The drawing under review shows one solid part. Ordinate dimensions are in mm from its lowest x, y, z. A direction names the side the tool comes from. Give positions to 0.01 mm unless a question says otherwise; leave off trailing zeros. Order: outer loops, then holes, each group sorted by start corner. A loop starts at its lowest first (then second) coordinate and runs counter-clockwise, first axis right, second up. Notation, with made-up numbers: (65, -16) - (95, -16) arc R20 ccw to (95, 5) - close; hole circle Ø6 at (53.25, -27.5). An arc over 180 degrees is marked (long way). Answer as a JSON object with one key per item and string values. Group by question number.
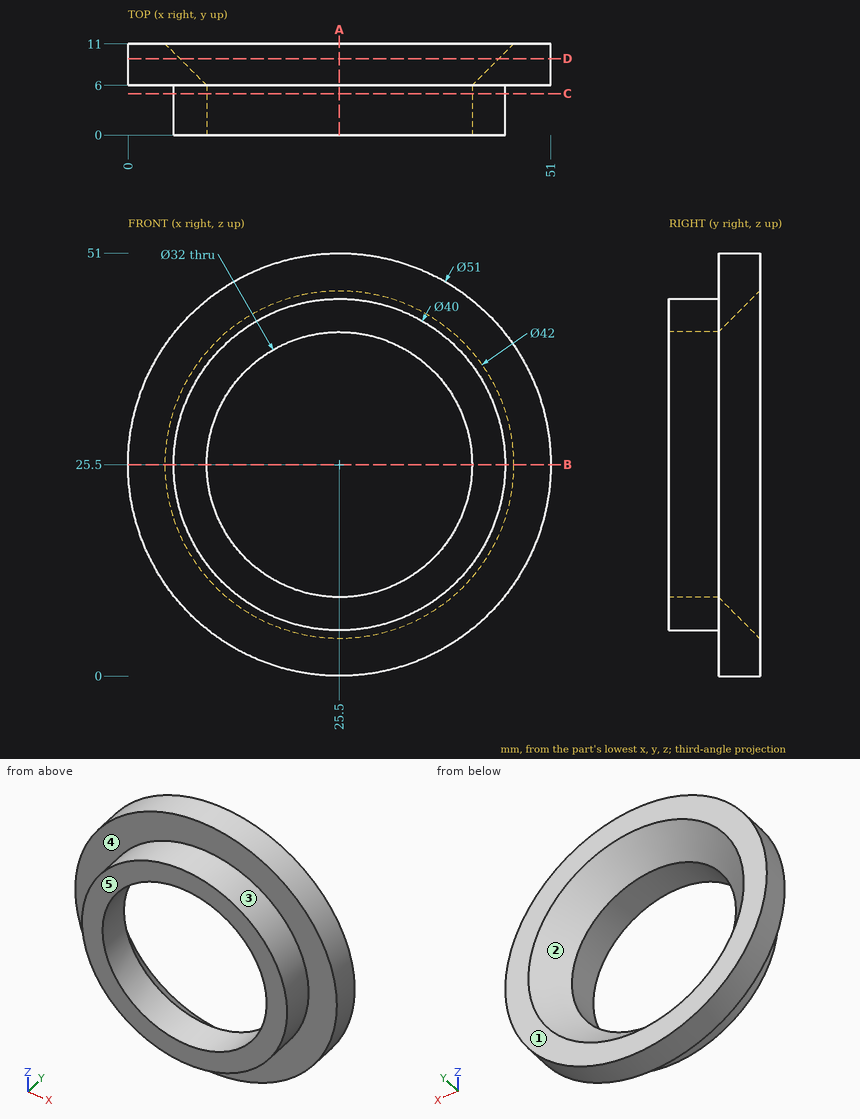
1) Consider section A-A (x = 25.5). Give the boundary of the cut face in (y, z), plus the area to 3 significant figures.
2) For line 1 (X direction, y = 1.9, z = 25.5); line 2 (Z direction, x = 14, y = 3.25), list the stretches that pass through material, from the lowest coordinate up.
3) Consider section C-C (y = 5). Give the boundary of the cut face in (x, z).
4) Mouldability with a two-part tool opening along X and no side actions: class the marked faces 1, 2 and 3 as released by +X, released by -X, zero draft, split by the parting line, or undercut.
5) For the marked faces 4 and 5, list the 3-axis set-ups (+Z, -Z, +X, -X, +Y, -Y) from which the entire face can be reached by the end or side of a thin tool; tool diameter is ignored.
6) For pin 1 (5 mm diameter, centred on x = 19, y = 1.5, fed in from -Z); pin 2 (6 mm diameter, centred on x = 11, z = 32.5, fed in from +Y), all flat-tipped, find the tip position at first contact; note any pin that passes through.
7) Consider section D-D (y = 9.25). Give the boundary of the cut face in (x, z).
8) Consider section B-B (z = 25.5). Give the boundary of the cut face in (x, y).
Result set:
{
 "1": {"outline": "(0, 5.5) - (6, 5.5) - (6, 0) - (11, 0) - (11, 4.5) - (6, 9.5) - (0, 9.5) - close; (0, 41.5) - (6, 41.5) - (11, 46.5) - (11, 51) - (6, 51) - (6, 45.5) - (0, 45.5) - close", "area": "118 mm2"},
 "2": {"line 1": "x = 5.5 to 9.5, 41.5 to 45.5", "line 2": "z = 9.14 to 14.38, 36.62 to 41.86"},
 "3": {"outline": "circle Ø40 at (25.5, 25.5); hole circle Ø32 at (25.5, 25.5)"},
 "4": {"face 1": "zero draft", "face 2": "undercut", "face 3": "split by the parting line"},
 "5": {"face 4": "-Y", "face 5": "+Z, -Z, +X, -X, -Y"},
 "6": {"pin 1": "stops at z = 5.9", "pin 2": "stops at y = 9.1"},
 "7": {"outline": "circle Ø51 at (25.5, 25.5); hole circle Ø38.5 at (25.5, 25.5)"},
 "8": {"outline": "(0, 6) - (5.5, 6) - (5.5, 0) - (9.5, 0) - (9.5, 6) - (4.5, 11) - (0, 11) - close; (41.5, 0) - (45.5, 0) - (45.5, 6) - (51, 6) - (51, 11) - (46.5, 11) - (41.5, 6) - close"}
}
